Check sheet for the modelled part. Datum: model origin and axes. Units: mm. A direction names the side the tool comes from. Round coordinates to 2 decimals unless told otherwise and drop trailing zeros. Write each loop counter-clockwise with the first axis right and the second up, starting at its lowest first coordinate (ties: lowest second). Pieces come first, ordered by that corner, then holes. Notation, with made-up numbers: (21, 16) - (48, 16) arc R25 cw to (48, 54) - close; hole circle Ø1 at (-33, 5). An arc over 180 degrees is marked (long way). Use one line per item in the form item = value. Start each with the question number.
1) Section check C-C (x = -62). Record the boundary of the cut face in (y, z), then the cut area to 4 significant figures.
2) Draft check along X on faces 4 (the face through (61.163, 7.395, 2.51)), 5 (the face through (-106, 7, -27.687)), 6 (the face through (116.15, 7.4, 2.25)), 7 (the face through (-117.843, 7, 19)). Enter one of: +X half, -X half, draft (parallel to the pull), parting line (faces both ways), or undercut.
3) Section check B-B (x = 95). Record the boundary of the cut face in (y, z).
4) Section check A-A (z = 12.5). Record the boundary of the cut face in (x, y).
5) Section check D-D (x = -5). Record the boundary of the cut face in (y, z).
6) Gauge pin test, flat ends, axial feed: P1, Ø4, axis at x = 83.5, y = 9, coming from the +Z side; P2, Ø1.2, axis at x = -78.5, y = 10.5, coming from the -Z side; P3, Ø1.5, axis at x = -82.5, y = 5, coming from the +Z side. Record the tip position at first contact, or that the pin passes through.
7) Set-up check for faces 1 (the face through (-114.4, 5.9, 4.734)), 2 (the face through (-117.843, 7, -13)), 3 (the face through (-79, 7, 6.799)): record each of +Z, -Z, +X, -X, +Y, -Y from which the full face is reachable in a straight line by a thin tool's end or side.
8) Scan lines: probe 1 along X at (y, z) = (13.25, 1.5); probe 2 along X at (y, z) = (8, 9.5); probe 3 along X at (y, z) = (5, 0) (3 decimals). Record each from-to range of solid material in increasing order.
from build123d import *

# Parameters (mm, degrees)
SKETCH1_R               = 6
BOSS_EXTRUDE1_DEPTH     = 15
SKETCH2_R               = 4
CUT_EXTRUDE1_DEPTH      = 28.686687264
CUT_EXTRUDE1_DEPTH_BACK = 34.233997448
SKETCH3_W               = 25.445516604
SKETCH3_H               = 3.920684712
CUT_EXTRUDE2_DEPTH      = 16


with BuildPart() as part:
    # Sketch1 → Boss-Extrude1 (new body)
    with BuildSketch(Plane(origin=(0, 0, 0), x_dir=(1, 0, 0), z_dir=(0, 1, 0))):
        with BuildLine():
            Line((-92.842511891, 27.686687264), (92.157488109, 21.226344908))
            ThreePointArc((92.157488109, 21.226344908), (116.157488109, -2.773655092), (92.157488109, -26.773655092))
            Line((92.157488109, -26.773655092), (-92.842511891, -33.233997448))
            Line((-92.842511891, -33.233997448), (-117.842511891, -33.233997448))
            Line((-117.842511891, -33.233997448), (-117.842511891, 27.686687264))
            Line((-117.842511891, 27.686687264), (-92.842511891, 27.686687264))
        make_face()
        with Locations((67.157488109, -2.773655092)):
            Circle(SKETCH1_R, mode=Mode.SUBTRACT)
        with Locations((42.157488109, -2.773655092)):
            Circle(SKETCH1_R, mode=Mode.SUBTRACT)
        with Locations((92.157488109, -2.773655092)):
            Circle(SKETCH1_R, mode=Mode.SUBTRACT)
        with BuildLine():
            Line((-80.95546537, 1.251344908), (-77.042511891, 1.251344908))
            Line((-77.042511891, 1.251344908), (-77.042511891, -6.798655092))
            Line((-77.042511891, -6.798655092), (-80.95546537, -6.798655092))
            ThreePointArc((-80.95546537, -6.798655092), (-105.392511891, -2.773655092), (-80.95546537, 1.251344908))
        make_face(mode=Mode.SUBTRACT)
    extrude(amount=BOSS_EXTRUDE1_DEPTH)

    # Sketch2 → Cut-Extrude1 (cut, two sides)
    with BuildSketch(Plane(origin=(0.426421377, 0, 0), x_dir=(-1, 0, 0), z_dir=(0, 0, -1))) as cut_extrude1_sk:
        with Locations((110.888582208, 7.369250935)):
            Circle(SKETCH2_R)
    extrude(amount=CUT_EXTRUDE1_DEPTH, mode=Mode.SUBTRACT)
    extrude(cut_extrude1_sk.sketch, amount=-CUT_EXTRUDE1_DEPTH_BACK, mode=Mode.SUBTRACT)

    # Sketch3 → Cut-Extrude2 (cut, through all)
    with BuildSketch(Plane(origin=(0, 15, 0), x_dir=(1, 0, 0), z_dir=(0, 1, 0))):
        with Locations((-111.290746627, -2.773655092)):
            Rectangle(SKETCH3_W, SKETCH3_H)
    extrude(amount=-CUT_EXTRUDE2_DEPTH, mode=Mode.SUBTRACT)


solid = part.part
Results are:
q1.outline = (0, -26.61) - (15, -26.61) - (15, 32.16) - (0, 32.16) - close
q1.area = 881.5 mm²
q2.face_4 = undercut
q2.face_5 = draft
q2.face_6 = +X half
q2.face_7 = -X half
q3.outline = (0, -21.06) - (15, -21.06) - (15, -2.51) - (0, -2.51) - close; (0, 8.06) - (15, 8.06) - (15, 26.6) - (0, 26.6) - close
q4.outline = (-117.84, 0) - (-100.77, 0) - (-100.77, 15) - (-117.84, 15) - close; (-84.91, 0) - (114.1, 0) - (114.1, 15) - (-84.91, 15) - close; hole circle Ø8 at (-110.46, 7.37)
q5.outline = (0, -24.62) - (15, -24.62) - (15, 30.17) - (0, 30.17) - close
q6.P1 = 27.15
q6.P2 = -27.21
q6.P3 = 32.9
q7.face_1 = -X, +Y, -Y
q7.face_2 = +Z, -Z, -X, +Y, -Y
q7.face_3 = +Y, -Y
q8.probe_1 = -77.04 to 36.29, 48.02 to 61.29, 73.02 to 86.29, 98.02 to 116.12
q8.probe_2 = -117.84 to -114.41, -106.51 to -103.44, -82.25 to 115.2
q8.probe_3 = -117.843 to -113.685, -107.239 to -105.082, -77.043 to 36.837, 47.478 to 61.837, 72.478 to 86.837, 97.478 to 115.997
